The model under review builds one solid part; all positions refer to its coordinate system, in mm. A direction names the side the tool comes from. Coordinates: 2 decimals unless noted, no trailing zeros. Loops run counter-clockwise (first coordinate to the right, second up) from the corner with the lowest first, then second, coordinate; pieces in that order, holes last. Notation, with made-up numbers: M 81,-27 L 92,-27 A16 ccw 92,-7 Z; hole C -8.75,-26 d10. An arc over 180 degrees is marked long. Return JSON: item names as keys, results as strings.
```python
from build123d import *

# Parameters (mm, degrees)
CROQUIS1_R              = 3.5
SALIENTE_EXTRUIR1_DEPTH = 40
CROQUIS2_R              = 1.5
CORTAR_EXTRUIR1_DEPTH   = 15
CROQUIS3_R              = 2
CORTAR_EXTRUIR2_DEPTH   = 15
CROQUIS4_R              = 1.4
CORTAR_EXTRUIR3_DEPTH   = 4.5


with BuildPart() as part:
    # Croquis1 → Saliente-Extruir1 (new body)
    with BuildSketch(Plane.XY):
        Circle(CROQUIS1_R)
    extrude(amount=SALIENTE_EXTRUIR1_DEPTH)

    # Croquis2 → Cortar-Extruir1 (cut)
    with BuildSketch(Plane.XY.offset(40)):
        Circle(CROQUIS2_R)
    extrude(amount=-CORTAR_EXTRUIR1_DEPTH, mode=Mode.SUBTRACT)

    # Croquis3 → Cortar-Extruir2 (cut)
    with BuildSketch(Plane(origin=(0, 0, 0), x_dir=(-1, 0, 0), z_dir=(0, 0, -1))):
        Circle(CROQUIS3_R)
    extrude(amount=-CORTAR_EXTRUIR2_DEPTH, mode=Mode.SUBTRACT)

    # Croquis4 → Cortar-Extruir3 (cut, through all)
    with BuildSketch(Plane(origin=(0, 0, 0), x_dir=(1, 0, 0), z_dir=(0, 1, 0))):
        with Locations((0, -4)):
            Circle(CROQUIS4_R)
        with Locations((0, -36)):
            Circle(CROQUIS4_R)
    extrude(amount=-CORTAR_EXTRUIR3_DEPTH, mode=Mode.SUBTRACT)


solid = part.part
```
1. Add section A-A on x = 0. Give the boundary of the cut face in (y, z), plus the area to 3 significant figures.
Check values:
{"outline": "M -3.5,0 L -2,0 L -2,2.6 L -3.5,2.6 Z; M -3.5,5.4 L -2,5.4 L -2,15 L 2,15 L 2,0 L 3.5,0 L 3.5,40 L 1.5,40 L 1.5,25 L -1.5,25 L -1.5,34.6 L -3.5,34.6 Z; M -3.5,37.4 L -1.5,37.4 L -1.5,40 L -3.5,40 Z", "area": "165 mm²"}
2. Add section B-B on y = 0. Give the boundary of the cut face in (x, z).
Check values:
{"outline": "M -3.5,0 L -2,0 L -2,15 L 2,15 L 2,0 L 3.5,0 L 3.5,40 L 1.5,40 L 1.5,25 L -1.5,25 L -1.5,40 L -3.5,40 Z"}
3. Add section D-D on z = 11.5. Give the boundary of the cut face in (x, y), plus the area to 3 significant figures.
Check values:
{"outline": "C 0,0 d7; hole C 0,0 d4", "area": "25.9 mm²"}
4. Insertion check: pin 1 Ø0.9 at (x, y) = (0, 0.5) entering from +Z. The pin has a flat end and moves straight along its axis. Give the tip position at first contact, or say it passes through.
Check values:
{"pin 1": "z = 25"}
5. To check wall thickness, follow line 1 (Z direction, x = 0, y = -2.45); line 2 (Y direction, x = 0, z = 28.5); line 3 (Y direction, x = 0, z = 10.5). State the ranges of each line that lie inside material, in increasing order.
Check values:
{"line 1": "0 to 2.6, 5.4 to 34.6, 37.4 to 40", "line 2": "-3.5 to -1.5, 1.5 to 3.5", "line 3": "-3.5 to -2, 2 to 3.5"}
6. The part is to be moulded in two halves that separate along X. For faces 5 (the face through (0, 2, 7)), 6 (the face through (2, -2, 0)), 7 (the face through (3.233, -1.341, 19.72)), say which applies: released by +X, released by -X, zero draft, split by the parting line, or undercut.
Check values:
{"face 5": "undercut", "face 6": "zero draft", "face 7": "split by the parting line"}
7. Machinability: for faces 1 (the face through (0, 0, 15)), 2 (the face through (-1.4, -2.33, 35.94)), 3 (the face through (0, -2, 40)), 4 (the face through (-0.195, 1.487, 32.605)), which of the approach directions +Z, -Z, +X, -X, +Y, -Y give a long, thin tool a straight path to every point of the face, cutting with its end or side? Answer none if there is none.
Check values:
{"face 1": "-Z", "face 2": "-Y", "face 3": "+Z, +X, -X, +Y, -Y", "face 4": "+Z"}
8. Add section C-C on z = 38. Give the boundary of the cut face in (x, y).
Check values:
{"outline": "C 0,0 d7; hole C 0,0 d3"}
